from build123d import *

# Parameters (mm, degrees)
SKETCH1_W           = 195.25
SKETCH1_H           = 195.25
BOSS_EXTRUDE1_DEPTH = 4.75
SKETCH2_W           = 10
SKETCH2_H           = 4.75
SKETCH2_W_2         = 4.75
SKETCH2_H_2         = 10
BOSS_EXTRUDE2_DEPTH = 4.75
SKETCH3_W           = 3
SKETCH3_H           = 12
SKETCH3_W_2         = 5.5
SKETCH3_H_2         = 3
CUT_EXTRUDE1_DEPTH  = 4.75
CIRPATTERN1_COUNT   = 4
SKETCH4_R           = 2.15
SKETCH4_W           = 60.17
SKETCH4_H           = 60.01
CUT_EXTRUDE2_DEPTH  = 283.882594905


with BuildPart() as part:
    # Sketch1 → Boss-Extrude1 (new body)
    with BuildSketch(Plane(origin=(0, 0, 0), x_dir=(1, 0, 0), z_dir=(0, 1, 0))):
        with Locations((-97.625, 97.625)):
            Rectangle(SKETCH1_W, SKETCH1_H)
    extrude(amount=BOSS_EXTRUDE1_DEPTH)

    # Sketch2 → Boss-Extrude2 (add)
    with BuildSketch(Plane(origin=(0, 4.75, 0), x_dir=(1, 0, 0), z_dir=(0, 1, 0))):
        with Locations((-155.25, 197.625)):
            Rectangle(SKETCH2_W, SKETCH2_H)
        with Locations((-97.625, 197.625)):
            Rectangle(SKETCH2_W, SKETCH2_H)
        with Locations((-40, 197.625)):
            Rectangle(SKETCH2_W, SKETCH2_H)
        with Locations((2.375, 155.25)):
            Rectangle(SKETCH2_W_2, SKETCH2_H_2)
        with Locations((2.375, 97.625)):
            Rectangle(SKETCH2_W_2, SKETCH2_H_2)
        with Locations((2.375, 40)):
            Rectangle(SKETCH2_W_2, SKETCH2_H_2)
        with Locations((-40, -2.375)):
            Rectangle(SKETCH2_W, SKETCH2_H)
        with Locations((-97.625, -2.375)):
            Rectangle(SKETCH2_W, SKETCH2_H)
        with Locations((-155.25, -2.375)):
            Rectangle(SKETCH2_W, SKETCH2_H)
        with Locations((-197.625, 40)):
            Rectangle(SKETCH2_W_2, SKETCH2_H_2)
        with Locations((-197.625, 97.625)):
            Rectangle(SKETCH2_W_2, SKETCH2_H_2)
        with Locations((-197.625, 155.25)):
            Rectangle(SKETCH2_W_2, SKETCH2_H_2)
    extrude(amount=-BOSS_EXTRUDE2_DEPTH)

    # Sketch3 → Cut-Extrude1 (cut)
    with BuildSketch(Plane(origin=(0, 4.75, 0), x_dir=(1, 0, 0), z_dir=(0, 1, 0))):
        with Locations((-126.4375, 6)):
            Rectangle(SKETCH3_W, SKETCH3_H)
        with Locations((-126.4375, 6.5)):
            Rectangle(SKETCH3_W_2, SKETCH3_H_2)
        with Locations((-68.8125, 6)):
            Rectangle(SKETCH3_W, SKETCH3_H)
        with Locations((-68.8125, 6.5)):
            Rectangle(SKETCH3_W_2, SKETCH3_H_2)
    cut_extrude1 = extrude(amount=-CUT_EXTRUDE1_DEPTH, mode=Mode.SUBTRACT)

    # CirPattern1: Cut-Extrude1 ×4 about axis
    cirpattern1_axis = Axis((-97.625, 0, -97.831288278), (0, 1, 0))
    for i in range(1, CIRPATTERN1_COUNT):
        add(cut_extrude1.rotate(cirpattern1_axis, i * 360 / CIRPATTERN1_COUNT), mode=Mode.SUBTRACT)

    # Sketch4 → Cut-Extrude2 (cut, through all)
    with BuildSketch(Plane(origin=(0, 4.75, 0), x_dir=(1, 0, 0), z_dir=(0, 1, 0))):
        with Locations(Location((-111.595, 25.715, 0), (0, 0, 270))):
            Circle(SKETCH4_R)
        with Locations(Location((-65.875, 93.66, 0), (0, 0, 270))):
            Circle(SKETCH4_R)
        with Locations(Location((-135.09, 93.66, 0), (0, 0, 270))):
            Circle(SKETCH4_R)
        with Locations((-100.165, 60.005)):
            Rectangle(SKETCH4_W, SKETCH4_H)
        with BuildLine():
            Line((-152.75, 43), (-152.75, 28))
            ThreePointArc((-152.75, 28), (-155.25, 25.5), (-157.75, 28))
            Line((-157.75, 28), (-157.75, 43))
            ThreePointArc((-157.75, 43), (-155.25, 45.5), (-152.75, 43))
        make_face()
        with BuildLine():
            Line((-42.58, 43), (-42.58, 28))
            ThreePointArc((-42.58, 28), (-45.08, 25.5), (-47.58, 28))
            Line((-47.58, 28), (-47.58, 43))
            ThreePointArc((-47.58, 43), (-45.08, 45.5), (-42.58, 43))
        make_face()
        with BuildLine():
            Line((-42.58, 86.01), (-42.58, 71.01))
            ThreePointArc((-42.58, 71.01), (-45.08, 68.51), (-47.58, 71.01))
            Line((-47.58, 71.01), (-47.58, 86.01))
            ThreePointArc((-47.58, 86.01), (-45.08, 88.51), (-42.58, 86.01))
        make_face()
        with BuildLine():
            Line((-110.25, 120.01), (-95.25, 120.01))
            ThreePointArc((-95.25, 120.01), (-90.25, 115.01), (-95.25, 110.01))
            Line((-95.25, 110.01), (-110.25, 110.01))
            ThreePointArc((-110.25, 110.01), (-115.25, 115.01), (-110.25, 120.01))
        make_face()
        with BuildLine():
            Line((-152.75, 86.01), (-152.75, 71.01))
            ThreePointArc((-152.75, 71.01), (-155.25, 68.51), (-157.75, 71.01))
            Line((-157.75, 71.01), (-157.75, 86.01))
            ThreePointArc((-157.75, 86.01), (-155.25, 88.51), (-152.75, 86.01))
        make_face()
    extrude(amount=-CUT_EXTRUDE2_DEPTH, mode=Mode.SUBTRACT)


solid = part.part
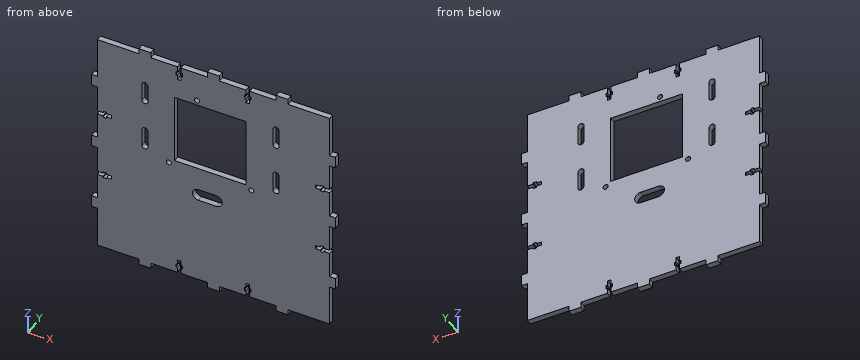
CAD build for the part. Positions are in the model's coordinates, mm. Round coordinates to 2 decimals unless told otherwise and drop trailing zeros. Loops run counter-clockwise (first coordinate to the right, second up) from the corner with the lowest first, then second, coordinate; pieces in that order, holes last. Notation, with made-up numbers: M 75.25,26 L 126.25,26 A22 ccw 126.25,63 Z; hole C 69.5,75 d3. An arc over 180 degrees is marked long. One line per question, with ' | ' between items. Start each with the question number.
Item 1: Cut at A-A, the plane z = -115.01. Write the cut outline in (x, y).
Item 2: Cut at B-B, the plane x = -118. Write the cut outline in (y, z).
Item 3: Cut at C-C, the plane y = 2.9. State how many separate pieces and enclosed holes the cut face has, plus the area to 3 significant figures.
Item 4: Wall check: line 1 (X direction, y = 2, z = -93.66) (3 decimals); line 2 (X direction, y = 2.3, z = -37.5); line 3 (X direction, y = 3.3, z = -10). Give the ranges that are in metal, low to high.
Item 5: Pin check, flat tips, straight feed: pin 1 Ø0.9 at (y, z) = (2.5, -69) entering from -X; pin 2 Ø2.5 at (y, z) = (3, -7) entering from +X; pin 3 Ø1.4 at (x, y) = (-66.5, 1.5) entering from -Z. Stop position of each tip, or through.
Item 6: Cut at D-D, the plane x = -17. Write the cut outline in (y, z), plus the area to 3 significant figures.
Responses:
1) outline: M -195.25,0 L -115.25,0 L -115.25,4.75 L -195.25,4.75 Z; M -90.25,0 L 0,0 L 0,4.75 L -90.25,4.75 Z
2) outline: M 0,-195.25 L 4.75,-195.25 L 4.75,-90.01 L 0,-90.01 Z; M 0,-30 L 4.75,-30 L 4.75,0 L 0,0 Z
3) separate pieces: 1 | enclosed holes: 9 | area: 34,100 mm²
4) line 1: x = -200 to -137.24, -132.94 to -68.025, -63.725 to 4.75 | line 2: x = -200 to -157.75, -152.75 to -130.25, -70.08 to -47.58, -42.58 to 4.75 | line 3: x = -195.25 to -127.94, -124.94 to -70.31, -67.31 to 0
5) pin 1: stops at x = -183.46 | pin 2: stops at x = 0 | pin 3: stops at z = -195.25
6) outline: M 0,-195.25 L 4.75,-195.25 L 4.75,0 L 0,0 Z | area: 927 mm²
